Autodesk Inventor part; units mm, degrees
ref_plane "YZ Plane" through (0, 0, 0) normal (1, 0, 0) x (0, 1, 0)
ref_plane "XZ Plane" through (0, 0, 0) normal (0, 1, 0) x (-1, 0, 0)
ref_plane "XY Plane" through (0, 0, 0) normal (0, 0, 1) x (1, 0, 0)
sketch "Sketch1" plane through (0, 0, 0) normal (0, 1, 0) x (-1, 0, 0)
  line L0 (0, 0) -> (-3.05, 0)
  line L1 (-3.05, 0) -> (-3.05, -7.62)
  line L2 (-3.05, -7.62) -> (0, -7.62)
  line L3 (0, -7.62) -> (0, 0)
  line L4 (0, 0) -> (-0.762, 0)
  line L5 (-0.762, 0) -> (-0.762, 13.208)
  line L6 (-0.762, 13.208) -> (0, 13.208)
  line L7 (0, 13.208) -> (0, 0)
  line L8 (-0.762, 13.208) -> (0, 16.0518)
  line L9 (-0.762, 13.208) -> (2.1821, 13.208) construction
  line L10 (0, 16.0518) -> (0, 13.208)
  dimension "d0" = 3.05
  dimension "d1" = 7.62
  dimension "d2" = 0.762
  dimension "d3" = 13.208
  dimension "d13" = 75
  dimension "d14" = 15
  dimension "d15" = 16.0518
  dimension "d16" = 23.6718
revolve "Revolution1" add sketch "Sketch1" angle 360 about axis through (0, 0, 13.208) along (0, 0, -1)
sketch "Sketch2" plane through (0, 0, -7.62) normal (0, 0, -1) x (-1, 0, 0)
  circle A0 centre (0, 0) radius 3.05
  circle A1 centre (0, 0) radius 1.5
  dimension "d5" = 3
extrude "Extrusion1" add sketch "Sketch2" along normal blind 4 contours A1
chamfer "Chamfer1" distance 1.143 angle 45 1 edges at (-3.05, 0, 0)
chamfer "Chamfer2" distance 0.254 angle 45 1 edges at (-3.05, 0, -7.62)
thread "Thread1"
properties part number "carbide_probe_30deg_tip_r01" material "Steel, High Strength, Low Alloy"
Here's how the part is built. I have some questions about the finished solid (model axes, mm). A direction names the side the tool comes from. Coordinates: 2 decimals unless noted, no trailing zeros. Loops run counter-clockwise (first coordinate to the right, second up) from the corner with the lowest first, then second, coordinate; pieces in that order, holes last. Notation, with made-up numbers: (51, -37) - (69, -37) arc R13 cw to (69, -28) - close; hole circle Ø2 at (56, 73.5). An arc over 180 degrees is marked (long way). Answer as CSV lines item,"result".
Q1. If we section it at A-A, the plane z = 10.75: Write out the boundary of the cut face in (x, y), and give its area (3 significant figures).
Response:
outline,"circle Ø1.52 at (0, 0)"
area,"1.82 mm2"
Q2. For faces 1 (the face through (0, 0, -11.62)), 2 (the face through (1.5, -0.07, -9.59)), 3 (the face through (0, 1, 0)), which set-ups out of +Z, -Z, +X, -X, +Y, -Y let a thin tool reach every point of the face, with its end or its side?
Response:
face 1,"-Z, +X, -X, +Y, -Y"
face 2,"-Z"
face 3,"+Z"
Q3. For pin 1 (3 mm diameter, centred on y = -2, z = 9, fed in from +X) (3 decimals); pin 2 (2 mm diameter, centred on y = 2, z = 10, fed in from -X), each with a flat end and sliding along its axis, tell me the tip position at first contact or that it passes through.
Response:
pin 1,"x = 0.575"
pin 2,"through"
Q4. If I drill on L1, parallel to X at y = 2.25, z = -6.5; L2, parallel to Z at x = 1.25, y = 0.25; L3, parallel to Y at x = 0.25, z = 9, over which ranges is the centre line in solid material (lowest first)? Write a range as [from, to].
Response:
L1,"[-2.06, 2.06]"
L2,"[-11.62, 0]"
L3,"[-0.72, 0.72]"
Q5. If we section it at B-B, the plane z = -4.75: Write out the boundary of the cut face in (x, y), and give its area (3 significant figures).
Response:
outline,"circle Ø6.1 at (0, 0)"
area,"29.2 mm2"
